Build history of the part. All positions in model axes, mm. A direction names the side the tool comes from. Round coordinates to 2 decimals unless told otherwise and drop trailing zeros. Write each loop counter-clockwise with the first axis right and the second up, starting at its lowest first coordinate (ties: lowest second). Pieces come first, ordered by that corner, then holes. Notation, with made-up numbers: (19.25, -6) -> (59.25, -6) arc R10 ccw to (59.25, 10) -> close; hole circle Ø5 at (-11, 52.25). An arc over 180 degrees is marked (long way). Answer as CSV lines item,"result".
from build123d import *

# Parameters (mm, degrees)
F1_DEPTH  = 25.4
F3_DEPTH  = 25.4
F5_DEPTH  = 29.718
F6_W      = 51.7507717013
F6_H      = 32.4542075396
F7_DEPTH  = 16.002
F9_DEPTH  = 9.652
F8_R      = 5.4354243812
F10_DEPTH = 9.906


with BuildPart() as f1:
    # F0 (on Front) → F1 (new body)
    with BuildSketch(Plane.XZ):
        with BuildLine():
            add(Edge.make_bspline(
                [(0, 0), (-7.2897283, -1.7897330566), (-14.8951404218, -1.670387598), (-22.8579116206, 0)],
                knots=[0.5519320833, 0.5519320833, 0.5519320833, 0.5519320833, 0.6673599665, 0.6673599665, 0.6673599665, 0.6673599665], degree=3))
            Line((0, 0), (-22.8579116206, 0))
        make_face()
        with BuildLine():
            Line((-22.8579116206, 0), (0, 0))
            Line((0, 0), (0, 44.5155379022))
            Line((0, 44.5155379022), (-101.6, 44.5155379022))
            add(Edge.make_bspline(
                [(-68.5272835275, 21.3313974768), (-78.9925734165, 28.0747606793), (-89.9973463161, 35.9700412347), (-101.6, 44.5155379022)],
                knots=[0.8708334463, 0.8708334463, 0.8708334463, 0.8708334463, 1, 1, 1, 1], degree=3))
            ThreePointArc((-68.5272835275, 21.3313974768), (-44.2668342264, 23.8746485463), (-31.3421689342, 3.1867159919))
            ThreePointArc((-31.3421689342, 3.1867159919), (-31.3463366195, 2.7486996352), (-31.3588381664, 2.3108418847))
            add(Edge.make_bspline(
                [(-22.8579116206, 0), (-25.647110234, 0.5851031828), (-28.4801553771, 1.3605130332), (-31.3588381664, 2.3108418847)],
                knots=[0.6673599665, 0.6673599665, 0.6673599665, 0.6673599665, 0.7077920326, 0.7077920326, 0.7077920326, 0.7077920326], degree=3))
        make_face()
        with BuildLine():
            Line((0, 44.5155379022), (0, 0))
            add(Edge.make_bspline(
                [(0, 44.5155379022), (23.3214331824, 41.0351589113), (49.3703629345, 35.9724451619), (18.3038264824, 4.4938524413), (0, 0)],
                knots=[0, 0, 0, 0, 0.2621034562, 0.5519320833, 0.5519320833, 0.5519320833, 0.5519320833], degree=3))
        make_face()
        with BuildLine():
            Line((-31.5638137301, 0), (-22.8579116206, 0))
            add(Edge.make_bspline(
                [(-22.8579116206, 0), (-25.647110234, 0.5851031828), (-28.4801553771, 1.3605130332), (-31.3588381664, 2.3108418847)],
                knots=[0.6673599665, 0.6673599665, 0.6673599665, 0.6673599665, 0.7077920326, 0.7077920326, 0.7077920326, 0.7077920326], degree=3))
            ThreePointArc((-31.3588381664, 2.3108418847), (-31.4321964371, 1.1528371057), (-31.5638137301, 0))
        make_face()
        with BuildLine():
            ThreePointArc((-77.1594360048, 0), (-54.3616248675, -19.8327399414), (-31.5638137301, 0))
            Line((-31.5638137301, 0), (-77.1594360048, 0))
        make_face()
        with BuildLine():
            Line((-77.1594360048, 0), (-31.5638137301, 0))
            ThreePointArc((-31.5638137301, 0), (-31.4321964371, 1.1528371057), (-31.3588381664, 2.3108418847))
            add(Edge.make_bspline(
                [(-31.3588381664, 2.3108418847), (-42.967062935, 6.1430219892), (-55.3173959076, 12.819538653), (-68.5272835275, 21.3313974768)],
                knots=[0.7077920326, 0.7077920326, 0.7077920326, 0.7077920326, 0.8708334463, 0.8708334463, 0.8708334463, 0.8708334463], degree=3))
            ThreePointArc((-68.5272835275, 21.3313974768), (-75.7001265591, 11.8217433237), (-77.1594360048, 0))
        make_face()
        with BuildLine():
            add(Edge.make_bspline(
                [(-68.5272835275, 21.3313974768), (-78.9925734165, 28.0747606793), (-89.9973463161, 35.9700412347), (-101.6, 44.5155379022)],
                knots=[0.8708334463, 0.8708334463, 0.8708334463, 0.8708334463, 1, 1, 1, 1], degree=3))
            Line((-101.6, 44.5155379022), (-101.6, 0))
            Line((-101.6, 0), (-77.1594360048, 0))
            ThreePointArc((-77.1594360048, 0), (-75.7001265591, 11.8217433237), (-68.5272835275, 21.3313974768))
        make_face()
        with BuildLine():
            Line((-101.6, 0), (-101.6, 44.5155379022))
            add(Edge.make_bspline(
                [(-134.6727164725, 21.3313974768), (-124.2074265835, 28.0747606793), (-113.2026536839, 35.9700412347), (-101.6, 44.5155379022)],
                knots=[0.8708334463, 0.8708334463, 0.8708334463, 0.8708334463, 1, 1, 1, 1], degree=3))
            ThreePointArc((-134.6727164725, 21.3313974768), (-128.1504425781, 13.2815066329), (-125.8189191992, 3.1867159919))
            ThreePointArc((-125.8189191992, 3.1867159919), (-125.8743972507, 1.5895086456), (-126.0405639952, 0))
            Line((-126.0405639952, 0), (-101.6, 0))
        make_face()
        with BuildLine():
            add(Edge.make_bspline(
                [(-134.6727164725, 21.3313974768), (-124.2074265835, 28.0747606793), (-113.2026536839, 35.9700412347), (-101.6, 44.5155379022)],
                knots=[0.8708334463, 0.8708334463, 0.8708334463, 0.8708334463, 1, 1, 1, 1], degree=3))
            Line((-101.6, 44.5155379022), (-203.2, 44.5155379022))
            add(Edge.make_bspline(
                [(-203.2, 44.5155379022), (-226.5214331824, 41.0351589113), (-252.5703629345, 35.9724451619), (-221.5038264824, 4.4938524413), (-203.2, 0)],
                knots=[0, 0, 0, 0, 0.2621034562, 0.5519320833, 0.5519320833, 0.5519320833, 0.5519320833], degree=3))
            Line((-203.2, 0), (-180.3420883794, 0))
            add(Edge.make_bspline(
                [(-180.3420883794, 0), (-177.552889766, 0.5851031828), (-174.7198446229, 1.3605130332), (-171.8411618336, 2.3108418847)],
                knots=[0.6673599665, 0.6673599665, 0.6673599665, 0.6673599665, 0.7077920326, 0.7077920326, 0.7077920326, 0.7077920326], degree=3))
            ThreePointArc((-171.8411618336, 2.3108418847), (-159.3249900183, 23.6788183658), (-134.6727164725, 21.3313974768))
        make_face()
        with BuildLine():
            ThreePointArc((-125.8189191992, 3.1867159919), (-128.1504425781, 13.2815066329), (-134.6727164725, 21.3313974768))
            add(Edge.make_bspline(
                [(-171.8411618336, 2.3108418847), (-160.232937065, 6.1430219892), (-147.8826040924, 12.819538653), (-134.6727164725, 21.3313974768)],
                knots=[0.7077920326, 0.7077920326, 0.7077920326, 0.7077920326, 0.8708334463, 0.8708334463, 0.8708334463, 0.8708334463], degree=3))
            ThreePointArc((-171.8411618336, 2.3108418847), (-171.7678035629, 1.1528371057), (-171.6361862699, 0))
            Line((-171.6361862699, 0), (-126.0405639952, 0))
            ThreePointArc((-126.0405639952, 0), (-125.8743972507, 1.5895086456), (-125.8189191992, 3.1867159919))
        make_face()
        with BuildLine():
            ThreePointArc((-171.6361862699, 0), (-148.8383751325, -19.8327399414), (-126.0405639952, 0))
            Line((-126.0405639952, 0), (-171.6361862699, 0))
        make_face()
        with BuildLine():
            ThreePointArc((-171.6361862699, 0), (-171.7678035629, 1.1528371057), (-171.8411618336, 2.3108418847))
            add(Edge.make_bspline(
                [(-180.3420883794, 0), (-177.552889766, 0.5851031828), (-174.7198446229, 1.3605130332), (-171.8411618336, 2.3108418847)],
                knots=[0.6673599665, 0.6673599665, 0.6673599665, 0.6673599665, 0.7077920326, 0.7077920326, 0.7077920326, 0.7077920326], degree=3))
            Line((-180.3420883794, 0), (-171.6361862699, 0))
        make_face()
        with BuildLine():
            Line((-180.3420883794, 0), (-203.2, 0))
            add(Edge.make_bspline(
                [(-203.2, 0), (-195.9102717, -1.7897330566), (-188.3048595782, -1.670387598), (-180.3420883794, 0)],
                knots=[0.5519320833, 0.5519320833, 0.5519320833, 0.5519320833, 0.6673599665, 0.6673599665, 0.6673599665, 0.6673599665], degree=3))
        make_face()
    extrude(amount=F1_DEPTH)

    # F2 (on face) → F3 (join)
    with BuildSketch(Plane.XY.offset(44.5155379022)):
        Polygon((-106.8298220634, -25.4), (-106.8298220634, 0), (-161.563180387, 0), align=None)
        Polygon((-52.0964637399, 0), (-106.8298220634, 0), (-106.8298220634, -25.4), align=None)
    extrude(amount=F3_DEPTH)

    # F4 (on face) → F5 (join)
    with BuildSketch(Plane(origin=(0, 0, 0), x_dir=(-1, 0, 0), z_dir=(0, 1, 0))):
        with BuildLine():
            ThreePointArc((120.0825944543, 47.0518544316), (115.8076187762, 57.3725586924), (105.4869145155, 61.6475343704))
            ThreePointArc((105.4869145155, 61.6475343704), (95.1662102547, 36.7311501709), (120.0825944543, 47.0518544316))
        make_face()
    extrude(amount=F5_DEPTH)

    # F6 (on face) → F7 (join)
    with BuildSketch(Plane(origin=(0, 0, 0), x_dir=(-1, 0, 0), z_dir=(0, 1, 0))):
        with Locations((108.4294952452, 45.8226948977)):
            Rectangle(F6_W, F6_H)
    extrude(amount=F7_DEPTH)

    # F8 (on face) → F9 (join)
    with BuildSketch(Plane(origin=(0, 16.002, 0), x_dir=(-1, 0, 0), z_dir=(0, 1, 0))):
        Polygon((128.5798549652, 57.735029608), (122.539177537, 57.4203245342), (122.539177537, 48.4996959567), (128.5798549652, 48.4996959567), align=None)
    extrude(amount=F9_DEPTH)

    # F8 (on face) → F10 (join)
    with BuildSketch(Plane(origin=(0, 16.002, 0), x_dir=(-1, 0, 0), z_dir=(0, 1, 0))):
        with Locations((124.7914806008, 38.2719635963)):
            Circle(F8_R)
    extrude(amount=F10_DEPTH)


solid = f1.part
1. Cut at B-B, the plane y = -5.5. Count the separate pieces of the cut face and the enclosed holes in it, then the cut area to 3 significant figures.
Results found:
separate pieces,"1"
enclosed holes,"2"
area,"14,000 mm2"
2. Probe line 1 along X through (y, z) = (-15.5, 15.5); line 2 along Y through (x, z) = (-61, -4); line 3 along X through (y, z) = (-16, 21.5). List the from-to ranges inside material, lowest first.
Results found:
line 1,"x = -229.68 to -168.29, -144.09 to -59.11, -34.91 to 26.48"
line 2,"y = -25.4 to 0"
line 3,"x = -234.7 to -162.79, -134.89 to -68.31, -40.41 to 31.5"
3. Mould opens along X. For faces 6 (the cylindrical face through (-149.3, -12.52, -19.83)), 7 (the flat face through (-108, 8, 29.596)), 8 (the flat face through (-79.85, -12.88, 57.04)), 9 (the flat face through (-27, -13, 0)) say: +X half, -X half, draft (parallel to the pull), parting line (faces both ways), or undercut.
Results found:
face 6,"undercut"
face 7,"draft"
face 8,"+X half"
face 9,"undercut"
4. Drop flat-ended pins along their axis: pin 1 Ø6.5 at (x, z) = (-125, 52.5) entering from +Y; pin 2 Ø1 at (y, z) = (16, 36.5) entering from -X; pin 3 Ø8.5 at (x, z) = (-123.5, 40) entering from +Y. Give the stop position or say it passes through.
Results found:
pin 1,"stops at y = 25.65"
pin 2,"stops at x = -134.3"
pin 3,"stops at y = 25.91"
5. Cut at A-A, the plane z = -9. Write the cut outline in (x, y), then the cut area to 3 significant figures.
Results found:
outline,"(-168.37, -25.4) -> (-129.31, -25.4) -> (-129.31, 0) -> (-168.37, 0) -> close; (-73.89, -25.4) -> (-34.83, -25.4) -> (-34.83, 0) -> (-73.89, 0) -> close"
area,"1,980 mm2"
6. Which spindle directions (+Z, -Z, +X, -X, +Y, -Y) get a long thin tool onto all of the face, cutting with end or side? Do faces 1 (the flat face through (-126, 21, 48.5)), 2 (the cylindrical face through (-124.08, 20.89, 43.66)), 3 (the flat face through (-41, -13, 44.516)), 4 (the flat face through (-128.58, 21, 53)), 5 (the flat face through (-122.539, 21, 53)). Say none if no direction does.
Results found:
face 1,"-X, +Y"
face 2,"+Y"
face 3,"+Z, +X, -Y"
face 4,"+Z, -X, +Y"
face 5,"+Z, +Y"
